Autodesk Inventor part; units mm, degrees
ref_plane "YZ Plane" through (0, 0, 0) normal (1, 0, 0) x (0, 1, 0)
ref_plane "XZ Plane" through (0, 0, 0) normal (0, 1, 0) x (-1, 0, 0)
ref_plane "XY Plane" through (0, 0, 0) normal (0, 0, 1) x (1, 0, 0)
sketch "Skizze1" plane through (0, 0, 0) normal (0, 1, 0) x (-1, 0, 0)
  line L0 (65, 5.2632) -> (0, 5.2632)
  line L1 (0, 5.2632) -> (0, -34.7368)
  line L2 (0, -34.7368) -> (20, -34.7368)
  line L3 (20, -34.7368) -> (20, 0.2632)
  line L4 (20, 0.2632) -> (65, 0.2632)
  line L5 (65, 0.2632) -> (65, 5.2632)
  point P0 (0, 0)
  dimension "d0" = 5
  dimension "d1" = 20
  dimension "d2" = 40
  dimension "d5" = 65
extrude "Extrusion1" add sketch "Skizze1" along normal blind 30
sketch "Skizze2" plane through (-65, 0, 5.2632) normal (0, 0, 1) x (1, 0, 0)
  line L0 (11, 9) -> (35, 9)
  line L1 (35, 9) -> (35, 21)
  line L2 (35, 21) -> (11, 21)
  line L3 (11, 21) -> (11, 9)
  line L4 (65, 0) -> (65, 30)
  line L5 (0, 30) -> (65, 30)
  dimension "d6" = 30
  dimension "d7" = 24
  dimension "d8" = 12
  dimension "d9" = 9
extrude "Extrusion2" cut sketch "Skizze2" against normal blind 5
sketch "Skizze3" plane through (0, 0, 5.2632) normal (1, 0, 0) x (0, 0, -1)
  circle A0 centre (10, 5) radius 1.7
  circle A1 centre (36, 5) radius 1.7
  circle A2 centre (10, 25) radius 1.7
  circle A3 centre (36, 25) radius 1.7
  line L0 (0, 0) -> (0, 30)
  line L1 (0, 30) -> (40, 30)
  line L2 (40, 0) -> (40, 30)
  point P0 (5.2632, 0)
  dimension "d12" = 3.4
  dimension "d13" = 3.4
  dimension "d14" = 3.4
  dimension "d15" = 3.4
  dimension "d16" = 10
  dimension "d17" = 20
  dimension "d18" = 5
  dimension "d19" = 10
  dimension "d20" = 4
  dimension "d21" = 20
  dimension "d22" = 4
  dimension "d23" = 5
extrude "Extrusion3" cut sketch "Skizze3" against normal blind 20
sketch "Skizze4" plane through (0, 0, 5.2632) normal (1, 0, 0) x (0, 0, -1)
  point P0 (5.2632, 0)
sketch "Skizze5" plane through (0, 0, -34.7368) normal (0, 0, -1) x (-1, 0, 0)
  arc A0 (0.0007, -11.0976) -> (-0.0008, 42.9427) centre (7.2057, 15.9227) ccw
  circle A1 centre (7.2057, 15.9227) radius 2.5
  point P0 (0, 0)
  dimension "d26" = 5
extrude "Extrusion4" cut sketch "Skizze5" against normal through all
properties part number "L-Halterung Servo"
Geometry check sheet. Reference: the model listing, model coordinates, mm. A direction names the side the tool comes from. Coordinates: 2 decimals unless noted, no trailing zeros. Loops run counter-clockwise (first coordinate to the right, second up) from the corner with the lowest first, then second, coordinate; pieces in that order, holes last. Notation, with made-up numbers: (36, -0.75) - (88, -0.75) arc R26 cw to (88, 22.25) - close; hole circle Ø4 at (-26.5, -8). An arc over 180 degrees is marked (long way). Use one line per item in the form item = value. Start each with the question number.
Item 1: Section check A-A, the plane x = -16. Enter the section's corners in (y, z), and give its area (3 significant figures).
Item 2: Gauge pin test, flat end, axial feed: pin 1 (9 mm diameter, centred on y = 12.5, z = -19.5, fed in from -X). Record the tip position at first contact, or that the pin passes through.
Item 3: Thickness scan on probe 1 along X at (y, z) = (25.25, -23.5); probe 2 along Z at (x, y) = (-30.5, 24.75); probe 3 along Z at (x, y) = (-3.5, 5.75). Record the ranges inside material, lowest first.
Item 4: Mould release check, pull along X, two halves, no side actions. Record for faces 1 (the face through (-65, 15, 3)), 2 (the face through (-42, 8, 0.263)), 3 (the face through (-30, 15, 3)): +X half, -X half, draft (parallel to the pull), parting line (faces both ways), or undercut.
Item 5: Section check B-B, the plane y = 11. Enter the section's corners in (x, z), and give its area (3 significant figures).
Item 6: Section check D-D, the plane x = -8. Enter the section's corners in (y, z), and give its area (3 significant figures).
Item 7: Tool access check on faces 4 (the face through (-20, 15, -17)), 5 (the face through (-18, 30, -10)), 6 (the face through (-42, 9, 3)). Record the directions out of +Z, -Z, +X, -X, +Y, -Y that give a thin tool (end or side, any length) a straight path to the whole face; none if there is none.
Item 8: Section check C-C, the plane y = 5. Enter the section's corners in (x, z).
Computed:
q1.outline = (0, -34.74) - (30, -34.74) - (30, 5.26) - (0, 5.26) - close; hole circle Ø3.4 at (5, -30.74); hole circle Ø3.4 at (5, -4.74); hole circle Ø3.4 at (25, -30.74); hole circle Ø3.4 at (25, -4.74)
q1.area = 1,160 mm2
q2.pin_1 = -20
q3.probe_1 = -20 to 0
q3.probe_2 = 0.26 to 5.26
q3.probe_3 = -34.74 to -32.26, -29.21 to -6.26, -3.21 to 5.26
q4.face_1 = -X half
q4.face_2 = draft
q4.face_3 = undercut
q5.outline = (-65, 0.26) - (-54, 0.26) - (-54, 5.26) - (-65, 5.26) - close; (-30, 0.26) - (-20, 0.26) - (-20, -34.74) - (0, -34.74) - (0, 5.26) - (-30, 5.26) - close
q5.area = 905 mm2
q6.outline = (0, -34.74) - (13.55, -34.74) - (13.55, 5.26) - (0, 5.26) - close; (18.29, -34.74) - (30, -34.74) - (30, 5.26) - (18.29, 5.26) - close; hole circle Ø3.4 at (5, -30.74); hole circle Ø3.4 at (5, -4.74); hole circle Ø3.4 at (25, -30.74); hole circle Ø3.4 at (25, -4.74)
q6.area = 974 mm2
q7.face_4 = -Z, -X, +Y, -Y
q7.face_5 = +Z, -Z, +X, -X, +Y
q7.face_6 = +Z, -Z
q8.outline = (-65, 0.26) - (-20, 0.26) - (-20, -3.04) - (0, -3.04) - (0, 5.26) - (-65, 5.26) - close; (-20, -34.74) - (0, -34.74) - (0, -32.44) - (-20, -32.44) - close; (-20, -29.04) - (0, -29.04) - (0, -6.44) - (-20, -6.44) - close
